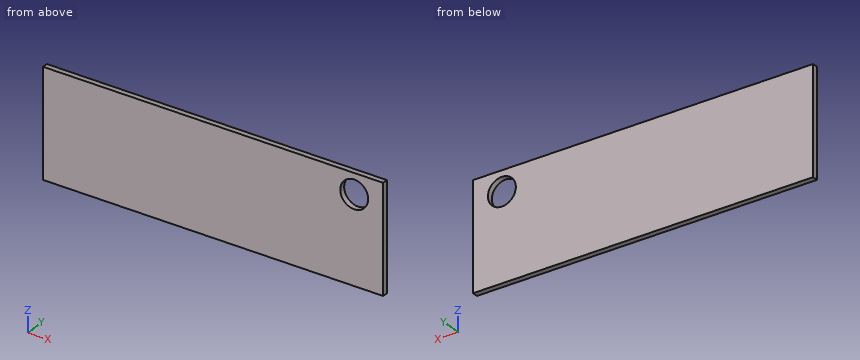
from build123d import *

# Parameters (mm, degrees)
F0_W           = 122.0296397805
F0_H           = 37.9903614521
F3_DEPTH       = 2
F5_D           = 10
F5_CBORE_D     = 10.0076
F5_CBORE_DEPTH = 5


# Not quite as in the source:
# - the program builds the solid bodies; features that only make, move or delete a surface that nothing else refers to are left out


with BuildPart() as f3:
    # F0 (on Front) → F3 (new body)
    with BuildSketch(Plane.XZ):
        Rectangle(F0_W, F0_H)
    extrude(amount=F3_DEPTH)

    # F5 (through all)
    with Locations(Plane(origin=(0, 0, 0), x_dir=(1, 0, 0), z_dir=(0, 1, 0))):
        with Locations((50.6538115442, -11.8000358343)):
            CounterBoreHole(F5_D / 2, F5_CBORE_D / 2, F5_CBORE_DEPTH)


solid = f3.part
Input: part model. Units: mm. Frame: model coordinates. Round coordinates to 2 decimals unless told otherwise and drop trailing zeros. Loops run counter-clockwise (first coordinate to the right, second up) from the corner with the lowest first, then second, coordinate; pieces in that order, holes last. Notation, with made-up numbers: M -26,1 L 3,1 A30 cw 3,30 Z; hole C 53,36 d1. An arc over 180 degrees is marked long. Answer as CSV lines item,"result". Start each with the question number.
(1) Section B-B, the plane z = 14. Output: boundary loops of the cut face in (x, y), plus the area to 3 significant figures.
(2) Section A-A, the plane x = 49.5. Output: boundary loops of the cut face in (y, z), plus the area to 3 significant figures.
(3) Section C-C, the plane y = -0.9. Output: boundary loops of the cut face in (x, z).
(4) First-contact query: pin 1 (9 mm diameter, centred on x = 50.65, z = 11.8, fed in from -Y). Flat tip, straight axial feed; report the tip coordinate or a pass-through.
(5) Line query: line 1 (X direction, y = -0.3, z = 11.5). Output: solid intervals per line, ascending. Write a range as [from, to].
Values found:
1,outline,"M -61.01,-2 L 46.16,-2 L 46.16,0 L -61.01,0 Z; M 55.15,-2 L 61.01,-2 L 61.01,0 L 55.15,0 Z"
1,area,"226 mm²"
2,outline,"M -2,-19 L 0,-19 L 0,6.93 L -2,6.93 Z; M -2,16.67 L 0,16.67 L 0,19 L -2,19 Z"
2,area,"56.5 mm²"
3,outline,"M -61.01,-19 L 61.01,-19 L 61.01,19 L -61.01,19 Z; hole C 50.65,11.8 d10.01"
4,pin 1,"passes through"
5,line 1,"x = [-61.01, 45.66], [55.65, 61.01]"
